Autodesk Inventor part; units mm, degrees
ref_plane "YZ Plane" through (0, 0, 0) normal (1, 0, 0) x (0, 1, 0)
ref_plane "XZ Plane" through (0, 0, 0) normal (0, 1, 0) x (-1, 0, 0)
ref_plane "XY Plane" through (0, 0, 0) normal (0, 0, 1) x (1, 0, 0)
sketch "Náčrt2" plane through (0, 0, 0) normal (0, 1, 0) x (-1, 0, 0)
  line L0 (30, 17.5) -> (-30, 17.5)
  line L1 (-30, 17.5) -> (-30, -17.5)
  line L2 (-30, -17.5) -> (30, -17.5)
  line L3 (30, -17.5) -> (30, 17.5)
  circle A0 centre (0, 0) radius 4
  point P0 (30, 0)
  point P1 (0, 17.5)
  dimension "d0" = 60
  dimension "d1" = 35
  dimension "d22" = 8
extrude "Vysunutí1" add sketch "Náčrt2" along normal blind 2.5
sketch "Náčrt5" plane through (-30, 0, -17.5) normal (-1, 0, 0) x (0, -1, 0)
  line L0 (0, 35) -> (0, 0)
  line L1 (0, 0) -> (20, 0)
  line L2 (20, 0) -> (20, 35)
  line L3 (20, 35) -> (0, 35)
edge flange "Obruba2" height 22.5 angle 90 thickness 2.5 bend radius 2.5 thickness toward (-1, 0, 0) relief tear relief width 2.5 relief depth 1.25 corner gap 2.5 corner form 0 edges at (-30, 0, 0) (30, 0, 0) wall of the first edge with corners at (-30, 0, 17.5) (-30, 0, -17.5) (-30, -20, -17.5) (-30, -20, 17.5)
bend "Ohyb2"
corner "Roh2"
equation "\"d29\" = ŠířkaVýštipu"
equation "\"d30\" = HloubkaVýštipu"
equation "\"d31\" = MinimálníZbytek"
equation "\"d32\" = PoloměrOhybu"
equation "\"d35\" = PoloměrOhybu"
equation "\"d36\" = VelikostRohovéhoVýštipu"
equation "\"d37\" = VelikostMezery"
equation "\"d38\" = VelikostJacobihoPoloměru"
equation "\"PoloměrOhybu\" = Tloušťka"
equation "\"ŠířkaVýštipu\" = Tloušťka"
equation "\"HloubkaVýštipu\" = 0.5 * Tloušťka"
equation "\"MinimálníZbytek\" = 2 * Tloušťka"
equation "\"PřechodovýPoloměr\" = PoloměrOhybu"
equation "\"VelikostJacobihoPoloměru\" = PoloměrOhybu"
equation "\"VelikostMezery\" = Tloušťka"
properties part number "DD_KVD_004_04_A" material "Nerezová ocel"
CAD build for the part. Positions are in the model's coordinates, mm. A direction names the side the tool comes from. Give positions to 0.01 mm unless a question says otherwise; leave off trailing zeros. Order: outer loops, then holes, each group sorted by start corner. A loop starts at its lowest first (then second) coordinate and runs counter-clockwise, first axis right, second up. Notation, with made-up numbers: M -15,-21 L 37,-21 A21 ccw 37,-9 Z; hole C 85.5,-35 d7. An arc over 180 degrees is marked long. Put each result on its own line as item: value. Start each with the question number.
(1) Saw through at B-B, the plane y = -9.5. Write the cut outline in (x, z).
(2) Saw through at D-D, the plane z = -11. Write the cut outline in (x, y).
(3) Which spindle directions (+Z, -Z, +X, -X, +Y, -Y) get a long thin tool onto all of the face, cutting with end or side? Do faces 4 (the flat face through (-32.5, -11, 0)), 5 (the cylindrical face through (-29.287, -0.752, -0.245)). Say none if no direction does.
(4) Mould opens along Z. For faces 1 (the cylindrical face through (31.07, 1, 0.25)), 2 (the cylindrical face through (0.867, 1.232, 3.905)), 3 (the flat face through (-0.2, 0.4, 17.5)) say: +Z half, -Z half, draft (parallel to the pull), parting line (faces both ways), or undercut.
(5) Saw through at A-A, the plane z = 0. Write the cut outline in (x, y), then the cut area to 3 significant figures.
(6) Flat gauge pins, fed straight in: pin 1 Ø6 at (y, z) = (-1, -5) entering from +X; pin 2 Ø8 at (x, z) = (-20, -4.5) entering from -Y. Where does each tip first touch, or does it go through?
(7) Drill centre lines: line 1 along Z through (x, y) = (0, 1.7); line 2 along X through (y, z) = (-6, 10); line 3 along Y through (x, z) = (18, -8.5). Where is each one in solid material? Low to high.
(8) Saw through at C-C, the plane x = 0. Write the cut outline in (y, z), then the cut area to 3 significant figures.
Check result:
1. outline: M -32.5,-17.5 L -30,-17.5 L -30,17.5 L -32.5,17.5 Z; M 30,-17.5 L 32.5,-17.5 L 32.5,17.5 L 30,17.5 Z
2. outline: M -32.5,-20 L -30,-20 L -30,-2.5 A2.5 cw -27.5,0 L 27.5,0 A2.5 cw 30,-2.5 L 30,-20 L 32.5,-20 L 32.5,-2.5 A5 ccw 27.5,2.5 L -27.5,2.5 A5 ccw -32.5,-2.5 Z
3. face 4: +Z, -Z, -X, +Y, -Y
3. face 5: +Z, -Z, -Y
4. face 1: draft
4. face 2: undercut
4. face 3: +Z half
5. outline: M -32.5,-20 L -30,-20 L -30,-2.5 A2.5 cw -27.5,0 L -4,0 L -4,2.5 L -27.5,2.5 A5 ccw -32.5,-2.5 Z; M 4,0 L 27.5,0 A2.5 cw 30,-2.5 L 30,-20 L 32.5,-20 L 32.5,-2.5 A5 ccw 27.5,2.5 L 4,2.5 Z
5. area: 234 mm2
6. pin 1: stops at x = 32.5
6. pin 2: stops at y = 0
7. line 1: z = -17.5 to -4, 4 to 17.5
7. line 2: x = -32.5 to -30, 30 to 32.5
7. line 3: y = 0 to 2.5
8. outline: M 0,-17.5 L 2.5,-17.5 L 2.5,-4 L 0,-4 Z; M 0,4 L 2.5,4 L 2.5,17.5 L 0,17.5 Z
8. area: 67.5 mm2
